The listing builds one solid part. Answer for the finished solid, in the listing's coordinates (mm). A direction names the side the tool comes from. Give positions to 0.01 mm unless a question says otherwise; leave off trailing zeros. Order: outer loops, then holes, each group sorted by start corner. A loop starts at its lowest first (then second) coordinate and runs counter-clockwise, first axis right, second up. Notation, with made-up numbers: (-35, 53) - (19, 53) arc R9 cw to (19, 61) - close; hole circle Ø6 at (-6.75, -5.75). An arc over 180 degrees is marked (long way). Answer in a Markdown table with one row per item.
from build123d import *

# Parameters (mm, degrees)
SKETCH1_R           = 7.5
BOSS_EXTRUDE1_DEPTH = 8
CUT_EXTRUDE1_DEPTH  = 5
SKETCH3_R           = 5
SKETCH3_R_2         = 3.31
EXTRUDE_THIN1_DEPTH = 35


with BuildPart() as part:
    # Sketch1 → Boss-Extrude1 (new body)
    with BuildSketch(Plane(origin=(0, 0, 0), x_dir=(0, 0, -1), z_dir=(1, 0, 0))):
        Circle(SKETCH1_R)
    extrude(amount=BOSS_EXTRUDE1_DEPTH)

    # Sketch2 → Cut-Extrude1 (cut)
    with BuildSketch(Plane(origin=(8, 0, 0), x_dir=(0, 0, -1), z_dir=(1, 0, 0))):
        Polygon((0, -5.773502692), (5, -2.886751346), (5, 2.886751346), (0, 5.773502692), (-5, 2.886751346), (-5, -2.886751346), align=None)
    extrude(amount=-CUT_EXTRUDE1_DEPTH, mode=Mode.SUBTRACT)

    # Sketch3 → Extrude-Thin1 (add)
    with BuildSketch(Plane.ZY):
        Circle(SKETCH3_R)
        Circle(SKETCH3_R_2, mode=Mode.SUBTRACT)
    extrude(amount=EXTRUDE_THIN1_DEPTH)


solid = part.part
Item 1: Find section B-B on y = 0. Write down the section's boundary in (x, z).
Answer block:
| item | result |
|---|---|
| outline | (-35, -5) - (0, -5) - (0, -7.5) - (8, -7.5) - (8, -5) - (3, -5) - (3, 5) - (8, 5) - (8, 7.5) - (0, 7.5) - (0, 5) - (-35, 5) - (-35, 3.31) - (0, 3.31) - (0, -3.31) - (-35, -3.31) - close |
Item 2: Find section D-D on x = -31. Write down the section's boundary in (y, z).
Answer block:
| item | result |
|---|---|
| outline | circle Ø10 at (0, 0); hole circle Ø6.62 at (0, 0) |
Item 3: Find section A-A on x = 5. Write down the section's boundary in (y, z).
Answer block:
| item | result |
|---|---|
| outline | circle Ø15 at (0, 0); hole (-5.77, 0) - (-2.89, -5) - (2.89, -5) - (5.77, 0) - (2.89, 5) - (-2.89, 5) - close |
Item 4: Each of these flat-tipped pins is pushed along its axis until it touches: P1, Ø1, axis at x = -24, z = 3.5, coming from the +Y side; P2, Ø1.5, axis at x = -2.5, y = -3.5, coming from the -Z side; P3, Ø1, axis at x = -2, y = -3.5, coming from the +Z side. Where does it stop, or does it pass through?
Answer block:
| item | result |
|---|---|
| P1 | y = 4 |
| P2 | z = -4.18 |
| P3 | z = 4 |
Item 5: Determine the mould class of faces 4 (the face through (8, -5, 2)), 5 (the face through (5.535, -4.31, 2.535)), 6 (the face through (3.944, 0.33, 7.493)) for opening direction Z: pulls with the +Z half, pulls with the -Z half, needs draft (parallel to the pull), parting line crosses it, or undercut.
Answer block:
| item | result |
|---|---|
| face 4 | needs draft |
| face 5 | undercut |
| face 6 | parting line crosses it |
Item 6: Which of the six approach directions +Z, -Z, +X, -X, +Y, -Y give full straight-line access (tool end or side, diameter ignored) to faces 1 (the face through (-35, -3.3, -1.2)), 2 (the face through (6, 0, -5)), 3 (the face through (0, 0, 0))?
Answer block:
| item | result |
|---|---|
| face 1 | +Z, -Z, -X, +Y, -Y |
| face 2 | +X |
| face 3 | -X |
Item 7: Find section C-C on z = 0.75. Write down the section's boundary in (x, y), then the cut area to 3 significant figures.
Answer block:
| item | result |
|---|---|
| outline | (-35, -4.94) - (0, -4.94) - (0, -7.46) - (8, -7.46) - (8, -5.34) - (3, -5.34) - (3, 5.34) - (8, 5.34) - (8, 7.46) - (0, 7.46) - (0, 4.94) - (-35, 4.94) - (-35, 3.22) - (0, 3.22) - (0, -3.22) - (-35, -3.22) - close |
| area | 186 mm² |
Item 8: Consider line 1 (Y direction, x = -20.5, z = 0); line 2 (Z direction, x = -17.5, y = -0.25); line 3 (X direction, y = -3, z = -5.75). Determine where each line is inside the solid, lowest interval first.
Answer block:
| item | result |
|---|---|
| line 1 | -5 to -3.31, 3.31 to 5 |
| line 2 | -4.99 to -3.3, 3.3 to 4.99 |
| line 3 | 0 to 8 |
